```python
from build123d import *

# Parameters (mm, degrees)
BOSS_EXTRUDE1_DEPTH = 20
FILLET1_R           = 20


with BuildPart() as part:
    # Sketch1 → Boss-Extrude1 (new body)
    with BuildSketch(Plane.XY):
        Polygon((0, 0), (-125, 0), (-125, 100), (-21.537340336, 100), (13.563596678, 150.129333232), (75, 107.111100506), align=None)
    extrude(amount=BOSS_EXTRUDE1_DEPTH)

    # Fillet1
    fillet1_edges = [part.edges().sort_by_distance(p)[0] for p in [
        (0, 0, 10),
        (-125, 0, 10),
        (-125, 100, 10),
        (-21.537340336, 100, 10),
        (13.563596678, 150.129333232, 10),
        (75, 107.111100506, 10),
    ]]
    fillet(fillet1_edges, radius=FILLET1_R)


solid = part.part
```
The listing builds one solid part. Answer for the finished solid, in the listing's coordinates (mm). A direction names the side the tool comes from. Round coordinates to 2 decimals unless told otherwise and drop trailing zeros. Loops run counter-clockwise (first coordinate to the right, second up) from the corner with the lowest first, then second, coordinate; pieces in that order, holes last.
Q1. Section B-B, the plane x = -58 is taken. Determine the outline of the cut face in (y, z).
Q2. Section C-C, the plane y = 93.5 is taken. Determine the outline of the cut face in (x, z), then the cut area to 3 significant figures.
Q3. Section A-A, the plane z = 17.75 is taken. Determine the outline of the cut face in (x, y).
Q4. Given pin 1 Ø2 at (y, z) = (47, 13.5) entering from +X; pin 2 Ø10 at (x, z) = (-58.5, 11.5) entering from +Y; pin 3 Ø6 at (x, z) = (9, 13) entering from +Y; pin 4 Ø1.5 at (x, y) = (-24, 38) entering from -Z, each flat-ended and moving along its own axis, determine where each tip first touches the part or whether it passes through.
Q5. Which of the six approach directions +Z, -Z, +X, -X, +Y, -Y give full straight-line access (tool end or side, diameter ignored) to faces 1 (the face through (-1.296, 2.198, 10.14)), 2 (the face through (-69, 100, 10))?
Q6. Find the intervals of material crossed by line 1 (Y direction, x = -91.5, z = 4.75); line 2 (Y direction, x = 14.5, z = 5.25); line 3 (X direction, y = 124.5, z = 15.5), in increasing order.
Completed:
1. outline: (0, 0) - (100, 0) - (100, 20) - (0, 20) - close
2. outline: (-119.76, 0) - (65.15, 0) - (65.15, 20) - (-119.76, 20) - close
2. area: 3,700 mm2
3. outline: (-125, 20) arc R20 ccw to (-105, 0) - (-10.41, 0) arc R20 ccw to (5.97, 8.53) - (63.53, 90.73) arc R20 ccw to (58.62, 118.58) - (29.95, 138.66) arc R20 ccw to (2.09, 133.75) - (-15.57, 108.53) arc R20 cw to (-31.95, 100) - (-105, 100) arc R20 ccw to (-125, 80) - close
4. pin 1: stops at x = 33.61
4. pin 2: stops at y = 100
4. pin 3: stops at y = 141.2
4. pin 4: stops at z = 0
5. face 1: +Z, -Z, +X, -Y
5. face 2: +Z, -Z, -X, +Y
6. line 1: y = 0 to 100
6. line 2: y = 20.71 to 141.88
6. line 3: x = -4.38 to 50.17
